```python
from build123d import *
from OCP.BRepFilletAPI import BRepFilletAPI_MakeChamfer

# Parameters (mm, degrees)
SKETCH_1_R               = 5
EXTRUDE_1_DEPTH          = 2
EXTRUDE_2_DEPTH          = 20
EXTRUDE_2_DEPTH_BACK     = 2
SKETCH_2_R               = 25.8
SKETCH_2_R_2             = 23.8
SKETCH_3_R               = 1.45
CUT_EXTRUDE_2_DEPTH      = 2
SKETCH_4_R               = 23.8
SKETCH_4_R_2             = 1.45
EXTRUDE_3_DEPTH          = 1
SKETCH_5_R               = 3.05
SKETCH_5_R_2             = 1.45
CUT_EXTRUDE_3_DEPTH      = 1
CUT_EXTRUDE_5_REACH      = 62.647
CUT_EXTRUDE_5_END_RADIUS = 25.8
SKETCH_6_R               = 7.625
CUT_EXTRUDE_START        = -16
CUT_EXTRUDE_6_DEPTH      = 16
EXTRUDE_5_DEPTH          = 19
CHAMFER_1_SIZE           = 1
CHAMFER_1_SIZE2          = 0.755634891
SKETCH_9_R               = 5.12
EXTRUDE_6_DEPTH          = 19
EXTRUDE_START            = -19
SKETCH_11_R              = 1.2
EXTRUDE_7_DEPTH          = 19
CHAMFER_3_SIZE           = 7.761762605
CHAMFER_3_SIZE_2         = 10
SKETCH_13_R              = 1.2
CUT_EXTRUDE_7_DEPTH      = 19
CUT_EXTRUDE_START_2      = -10
CUT_EXTRUDE_8_DEPTH      = 10
SKETCH_15_R              = 5.12
CUT_EXTRUDE_9_DEPTH      = 10


with BuildPart() as part:
    # 草图1 → 凸台-拉伸1 (new body)
    with BuildSketch(Plane.XY):
        with BuildLine():
            ThreePointArc((64, 25.8), (38.2, 0), (64, -25.8))
            ThreePointArc((64, -25.8), (82.243354955, -18.243354955), (89.8, 0))
            ThreePointArc((89.8, 0), (82.243354955, 18.243354955), (64, 25.8))
        make_face()
        with Locations((64, 0)):
            Circle(SKETCH_1_R, mode=Mode.SUBTRACT)
    extrude(amount=EXTRUDE_1_DEPTH)

    # 草图2 → 凸台-拉伸2 (add, two sides: drawn at the far end of the back side and taken through both)
    with BuildSketch(Plane.XY.offset(2).offset(-EXTRUDE_2_DEPTH_BACK)):
        with Locations((64, 0)):
            Circle(SKETCH_2_R)
        with Locations((64, 0)):
            Circle(SKETCH_2_R_2, mode=Mode.SUBTRACT)
    extrude(amount=EXTRUDE_2_DEPTH + EXTRUDE_2_DEPTH_BACK)

    # 草图3 → 切除-拉伸2 (cut)
    with BuildSketch(Plane.XY.offset(2)):
        with Locations((64, -16.8)):
            Circle(SKETCH_3_R)
    extrude(amount=-CUT_EXTRUDE_2_DEPTH, mode=Mode.SUBTRACT)

    # 草图4 → 凸台-拉伸3 (add)
    with BuildSketch(Plane.XY.offset(2)):
        with Locations((64, 0)):
            Circle(SKETCH_4_R)
        with Locations((64, -16.8)):
            Circle(SKETCH_4_R_2, mode=Mode.SUBTRACT)
    extrude(amount=EXTRUDE_3_DEPTH)

    # 草图5 → 切除-拉伸3 (cut)
    with BuildSketch(Plane(origin=(0, 0, 0), x_dir=(-1, 0, 0), z_dir=(0, 0, -1))):
        with Locations((-64, -16.8)):
            Circle(SKETCH_5_R)
        with Locations(Location((-64, -16.8, 0), (0, 0, 180))):
            Circle(SKETCH_5_R_2, mode=Mode.SUBTRACT)
    extrude(amount=-CUT_EXTRUDE_3_DEPTH, mode=Mode.SUBTRACT)

    # 切除-拉伸5: up to this cylinder (the profile starts inside it)
    cut_extrude_5_end = Plane(origin=(64, 0, 12.5), z_dir=(0, 0, -1)) * Cylinder(CUT_EXTRUDE_5_END_RADIUS, 177.894, mode=Mode.PRIVATE)
    # 草图6 → 切除-拉伸5 (cut, up to the surface)
    with BuildSketch(Plane(origin=(74.5, -5.45, -15.2), x_dir=(0, 0, -1), z_dir=(0, 1, 0)), mode=Mode.PRIVATE) as cut_extrude_5_sk1:
        with Locations(Location((-27.7, 10.5, 0), (0, 0, 90))):
            Circle(SKETCH_6_R)
    cut_extrude_5_tool1 = extrude(cut_extrude_5_sk1.sketch, amount=-CUT_EXTRUDE_5_REACH, mode=Mode.PRIVATE) & cut_extrude_5_end
    add(cut_extrude_5_tool1.solids().sort_by_distance((64, -5.45, 12.5))[0], mode=Mode.SUBTRACT)

    # 草图7 → 切除-拉伸6 (cut)
    with BuildSketch(Plane.XY.offset(22).offset(CUT_EXTRUDE_START)):
        with BuildLine():
            ThreePointArc((48.798857294, -18.312980654), (47.30860295, -16.965767431), (45.937273528, -15.497674419))
            Line((45.937273528, -15.497674419), (44.419397354, -16.8))
            ThreePointArc((44.419397354, -16.8), (45.784957677, -18.271623715), (47.260809567, -19.632613266))
            Line((47.260809567, -19.632613266), (48.798857294, -18.312980654))
        make_face()
        with BuildLine():
            Line((44.419397354, -16.8), (45.937273528, -15.497674419))
            ThreePointArc((45.937273528, -15.497674419), (44.694639643, -13.919161667), (43.589554969, -12.241475957))
            Line((43.589554969, -12.241475957), (42.051507242, -13.561108569))
            ThreePointArc((42.051507242, -13.561108569), (43.172397024, -15.22665276), (44.419397354, -16.8))
        make_face()
        with BuildLine():
            Line((64, 25.8), (64, 23.8))
            ThreePointArc((64, 23.8), (66.007150396, 23.715213414), (68, 23.461457755))
            Line((68, 23.461457755), (68, 25.488036409))
            ThreePointArc((68, 25.488036409), (66.006073359, 25.721890865), (64, 25.8))
        make_face()
        with BuildLine():
            ThreePointArc((60, 23.461457755), (61.992849604, 23.715213414), (64, 23.8))
            Line((64, 23.8), (64, 25.8))
            ThreePointArc((64, 25.8), (61.993926641, 25.721890865), (60, 25.488036409))
            Line((60, 25.488036409), (60, 23.461457755))
        make_face()
    extrude(amount=CUT_EXTRUDE_6_DEPTH, mode=Mode.SUBTRACT)

    # 草图8 → 凸台-拉伸5 (add)
    with BuildSketch(Plane.XY.offset(3)):
        with BuildLine():
            Line((73.7, -20.16), (73.7, -21.733614518))
            ThreePointArc((73.7, -21.733614518), (76.567494222, -20.211335655), (79.201142706, -18.312980654))
            Line((79.201142706, -18.312980654), (73.7, -6.16))
            Line((73.7, -6.16), (73.7, -20.16))
        make_face()
        with BuildLine():
            Line((54.3, -20.16), (54.3, -6.16))
            Line((54.3, -6.16), (48.798857294, -18.312980654))
            ThreePointArc((48.798857294, -18.312980654), (51.432505778, -20.211335655), (54.3, -21.733614518))
            Line((54.3, -21.733614518), (54.3, -20.16))
        make_face()
    extrude(amount=EXTRUDE_5_DEPTH)

    # 倒角1: one chamfer whose edges measure the first distance from different faces: ONE call of the kernel's chamfer builder (chamfer() names one face for all edges)
    chamfer_1_edges_1 = [part.edges().sort_by_distance(p)[0] for p in [
        (73.7, -6.16, 12.5),
    ]]
    chamfer_1_side_1 = [part.faces().sort_by_distance(p)[0] for p in [
        (76.450571353, -12.236490327, 12.5),
    ]]
    chamfer_1_edges_2 = [part.edges().sort_by_distance(p)[0] for p in [
        (54.3, -6.16, 12.5),
    ]]
    chamfer_1_side_2 = [part.faces().sort_by_distance(p)[0] for p in [
        (54.3, -13.946807259, 12.5),
    ]]
    chamfer_1 = BRepFilletAPI_MakeChamfer(part.part.solid().wrapped)
    for e in chamfer_1_edges_1:
        chamfer_1.Add(CHAMFER_1_SIZE, CHAMFER_1_SIZE2, e.wrapped, chamfer_1_side_1[0].wrapped)  # the first distance lies on this face
    for e in chamfer_1_edges_2:
        chamfer_1.Add(CHAMFER_1_SIZE, CHAMFER_1_SIZE2, e.wrapped, chamfer_1_side_2[0].wrapped)  # the first distance lies on this face
    add(Compound.cast(chamfer_1.Shape()), mode=Mode.REPLACE)

    # 草图9 → 凸台-拉伸6 (add)
    with BuildSketch(Plane.XY.offset(3)):
        with BuildLine():
            ThreePointArc((71.12, 0), (60.944269687, 6.430934011), (59.502889817, -5.52))
            Line((59.502889817, -5.52), (64, -5.52))
            Line((64, -5.52), (68.497110183, -5.52))
            ThreePointArc((68.497110183, -5.52), (70.430934011, -3.055730313), (71.12, 0))
        make_face()
        with Locations((64, 0)):
            Circle(SKETCH_9_R, mode=Mode.SUBTRACT)
    extrude(amount=EXTRUDE_6_DEPTH)

    # 草图11 → 凸台-拉伸7 (add)
    # profile 1 of 2: a face of its own
    with BuildSketch(Plane.XY.offset(22).offset(EXTRUDE_START)):
        with BuildLine():
            Line((74.1123773, 7.071013151), (79.201142706, 18.312980654))
            ThreePointArc((79.201142706, 18.312980654), (76.567494222, 20.211335655), (73.7, 21.733614518))
            Line((73.7, 21.733614518), (73.7, 6.915634891))
            Line((73.7, 6.915634891), (74.1123773, 7.071013151))
        make_face()
        with Locations((76.450571353, 18.312980654)):
            Circle(SKETCH_11_R, mode=Mode.SUBTRACT)
    # profile 2 of 2: a face of its own
    with BuildSketch(Plane.XY.offset(22).offset(EXTRUDE_START)):
        with BuildLine():
            ThreePointArc((54.3, 21.733614518), (51.432505778, 20.211335655), (48.798857294, 18.312980654))
            Line((48.798857294, 18.312980654), (53.988393324, 6.848393324))
            Line((53.988393324, 6.848393324), (54.3, 7.16))
            Line((54.3, 7.16), (54.3, 21.733614518))
        make_face()
        with Locations((51.549428647, 18.312980654)):
            Circle(SKETCH_11_R, mode=Mode.SUBTRACT)
    extrude(amount=EXTRUDE_7_DEPTH)

    # 倒角3
    # the kernel refuses this chamfer: 10, 7.761762605 mm, written as the material it takes off along each edge
    with BuildSketch(Plane(origin=(53.988393324, 6.848393324, 3), x_dir=(-0.45377895497770065, 0.8911142799996788, 0), z_dir=(0, 0, 1)), Plane(origin=(73.7, 6.915634891, 3), x_dir=(-0.045923294763777815, 0.9989449689537653, 0), z_dir=(0, 0, 1))) as chamfer_3_piece_1:
        Polygon((CHAMFER_3_SIZE * 0.998944968965, -CHAMFER_3_SIZE * 0.0459232947643), (CHAMFER_3_SIZE_2 * 0.309242773975, -CHAMFER_3_SIZE_2 * 0.950983126424), (0, 0), align=None)
    extrude(amount=44.71682988, mode=Mode.SUBTRACT)

    # 草图13 → 切除-拉伸7 (cut)
    with BuildSketch(Plane.XY.offset(22)):
        with Locations((76.450571353, -18.312980654)):
            Circle(SKETCH_13_R)
        with Locations((51.549428647, -18.312980654)):
            Circle(SKETCH_13_R)
    extrude(amount=-CUT_EXTRUDE_7_DEPTH, mode=Mode.SUBTRACT)

    # 草图14 → 切除-拉伸8 (cut)
    with BuildSketch(Plane.XY.offset(22).offset(CUT_EXTRUDE_START_2)):
        with BuildLine():
            Line((56.375, -22.54549567), (56.375, -24.647502409))
            ThreePointArc((56.375, -24.647502409), (64, -25.8), (71.625, -24.647502409))
            Line((71.625, -24.647502409), (71.625, -22.54549567))
            ThreePointArc((71.625, -22.54549567), (64, -23.8), (56.375, -22.54549567))
        make_face()
    extrude(amount=CUT_EXTRUDE_8_DEPTH, mode=Mode.SUBTRACT)

    # 草图15 → 切除-拉伸9 (cut)
    with BuildSketch(Plane.XY.offset(3).offset(CUT_EXTRUDE_START_2)):
        with Locations((64, 0)):
            Circle(SKETCH_15_R)
    extrude(amount=CUT_EXTRUDE_9_DEPTH, mode=Mode.SUBTRACT)


solid = part.part
```
Source: CAD feature listing. Evaluate the final solid. Frame: model axes, mm. A direction names the side the tool comes from. Coordinates: 2 decimals unless noted, no trailing zeros. Loops run counter-clockwise (first coordinate to the right, second up) from the corner with the lowest first, then second, coordinate; pieces in that order, holes last. Notation, with made-up numbers: (57.5, -0.75) -> (91.5, -0.75) arc R16 cw to (91.5, 27.25) -> close; hole circle Ø7 at (7.25, -22). An arc over 180 degrees is marked (long way). One line per item, written item: value. Start each with the question number.
Q1. Section query B-B, the plane z = 19.5. Give the number of separate pieces and of enclosed holes in the cut face, and give its area (3 significant figures).
Q2. Set-up query: faces 4 (the face through (43, 12, 22)), 5 (the face through (54.3, 18, 12)), 6 (the face through (69.4, 0.4, 0)), 7 (the face through (56.375, -24, 17)), 8 (the face through (67.047, -16.666, 0.493)). Return all of +Z, -Z, +X, -X, +Y, -Y with unobstructed straight access to the full face (end or side cutting, diameter ignored); none if empty.
Q3. Contact query for flat-ended pins moving along their axis: P1, Ø6, axis at y = -16.5, z = 17.5, coming from the -X side; P2, Ø7.5, axis at y = -16, z = 13, coming from the -X side; P3, Ø7, axis at x = 62.5, z = 10.5, coming from the -Y side; P4, Ø2.5, axis at x = 64, y = -16.8, coming from the -Z side. Output: stop coordinate, or through.
Q4. Section query A-A, the plane x = 64. Return the cut outline in (y, z) (3 decimals).
Q5. Mould query, pull axis Y, two halves, no side actions, for faces 1 (the face through (52, -17, 22)), 2 (the face through (52, -18, 3)), 3 (the face through (69, 6, 3)). Classes: pulls with the +Y half, pulls with the -Y half, needs draft (parallel to the pull), parting line crosses it, or undercut.
Q6. Line query: line 1 along X through (y, z) = (-11, 4.5); line 2 along X through (y, z) = (-18.5, 15); line 3 along Y through (x, z) = (65, 1.25). Output: solid intervals per line, ascending.
Q7. Section query C-C, the plane y = -8. Return the cut outline in (x, z).
Results:
1. separate pieces: 4
1. enclosed holes: 5
1. area: 445 mm^2
2. face 4: +Z, +X, -X, +Y, -Y
2. face 5: +Z
2. face 6: -Z, +X, -X, +Y, -Y
2. face 7: +Z, -Y
2. face 8: -Z
3. P1: x = 42.01
3. P2: x = 41.29
3. P3: y = -5.52
3. P4: through
4. outline: (-25.8, 0) -> (-19.85, 0) -> (-19.85, 1) -> (-18.25, 1) -> (-18.25, 3) -> (-23.8, 3) -> (-23.8, 4.875) -> (-25.8, 4.875) -> close; (-15.35, 1) -> (-13.75, 1) -> (-13.75, 0) -> (-5.12, 0) -> (-5.12, 22) -> (-5.52, 22) -> (-5.52, 3) -> (-15.35, 3) -> close; (5.12, 0) -> (25.8, 0) -> (25.8, 6) -> (23.8, 6) -> (23.8, 3) -> (7.12, 3) -> (7.12, 22) -> (5.12, 22) -> close
5. face 1: needs draft
5. face 2: undercut
5. face 3: undercut
6. line 1: 40.66 to 42.89, 52.11 to 54.3, 73.7 to 75.89, 85.11 to 87.34
6. line 2: 48.58 to 50.36, 52.73 to 54.3, 73.7 to 75.27, 77.64 to 81.98
6. line 3: -25.78 to -17.85, -15.75 to -5.02, 5.02 to 25.78
7. outline: (39.47, 0) -> (88.53, 0) -> (88.53, 22) -> (86.42, 22) -> (86.42, 3) -> (74.53, 3) -> (74.53, 22) -> (73.7, 22) -> (73.7, 3) -> (54.3, 3) -> (54.3, 22) -> (53.47, 22) -> (53.47, 3) -> (41.58, 3) -> (41.58, 22) -> (39.47, 22) -> close
